Autodesk Inventor part; units mm, degrees
ref_plane "YZ Plane" through (0, 0, 0) normal (1, 0, 0) x (0, 1, 0)
ref_plane "XZ Plane" through (0, 0, 0) normal (0, 1, 0) x (-1, 0, 0)
ref_plane "XY Plane" through (0, 0, 0) normal (0, 0, 1) x (1, 0, 0)
sketch "Sketch3" plane through (0, 0, 0) normal (0, 1, 0) x (-1, 0, 0)
  line L0 (0, 0) -> (25, 0)
  line L1 (25, 0) -> (25, -80)
  line L2 (25, -80) -> (0, -80)
  line L3 (0, -80) -> (0, 0)
  dimension "d21" = 25
  dimension "d22" = 80
extrude "Extrusion2" add sketch "Sketch3" along normal blind 1
sketch "Sketch4" plane through (0, 1, 0) normal (0, 1, 0) x (1, 0, 0)
  line L0 (-25, 80) -> (-25, 0) construction
  line L1 (-25, 40) -> (0, 40) construction
  line L2 (0, 0) -> (0, 80) construction
  point P0 (-5, 15.9)
  point P1 (-5, 64.1)
  dimension "d25" = 5
  dimension "d26" = 48.2
hole "Hole2" at (-5, 1, -15.9) at (-5, 1, -64.1) direction (0, -1, 0) diameter 3.4 end through all
properties part number "PCB"
Can you work these out from the model? Positions are in its coordinate system, mm. Round coordinates to 2 decimals unless told otherwise and drop trailing zeros. Loops run counter-clockwise (first coordinate to the right, second up) from the corner with the lowest first, then second, coordinate; pieces in that order, holes last. Notation, with made-up numbers: (57.5, 65) -> (116.5, 65) arc R17 cw to (116.5, 83) -> close; hole circle Ø7 at (-8, -3.5). An arc over 180 degrees is marked (long way). Answer in a Markdown table with one row per item.
Item 1: We'd pull the mould along X, two halves only. Please class faces 1 (the cylindrical face through (-5.07, 0.49, -65.8)), 2 (the flat face through (-12, 1, -39)), 3 (the cylindrical face through (-3.97, 0.49, -17.25)): released by +X, released by -X, zero draft, split by the parting line, or undercut.
Answer block:
| item | result |
|---|---|
| face 1 | undercut |
| face 2 | zero draft |
| face 3 | undercut |
Item 2: Suppose I cut it at A-A, the plane z = -64.1. List the corners of the cut face in (x, y) for me, plus the area to 3 significant figures.
Answer block:
| item | result |
|---|---|
| outline | (-25, 0) -> (-6.7, 0) -> (-6.7, 1) -> (-25, 1) -> close; (-3.3, 0) -> (0, 0) -> (0, 1) -> (-3.3, 1) -> close |
| area | 21.6 mm² |
Item 3: Suppose I cut it at B-B, the plane x = -5. List the corners of the cut face in (y, z) for me.
Answer block:
| item | result |
|---|---|
| outline | (0, -80) -> (1, -80) -> (1, -65.8) -> (0, -65.8) -> close; (0, -62.4) -> (1, -62.4) -> (1, -17.6) -> (0, -17.6) -> close; (0, -14.2) -> (1, -14.2) -> (1, 0) -> (0, 0) -> close |
Item 4: If I drill on probe 1 along Z at (x, y) = (-5, 0.4); probe 2 along X at (y, z) = (0.55, -64.1); probe 3 along Z at (x, y) = (-4.5, 0.2), over which ranges is the centre line in solid material (lowest first)?
Answer block:
| item | result |
|---|---|
| probe 1 | -80 to -65.8, -62.4 to -17.6, -14.2 to 0 |
| probe 2 | -25 to -6.7, -3.3 to 0 |
| probe 3 | -80 to -65.72, -62.48 to -17.52, -14.28 to 0 |
